```python
from build123d import *

# Parameters (mm, degrees)
ESBO_O1_R                = 2.95
RESSALTO_EXTRUS_O1_DEPTH = 16.15
RESSALTO_EXTRUS_O2_DEPTH = 32.3
FILETE1_R                = 1.5
ESBO_O3_R                = 3.25
CORTE_EXTRUS_O1_DEPTH    = 21.540435635
ESBO_O5_R                = 3.25
ESBO_O5_R_2              = 2.1
RESSALTO_EXTRUS_O3_DEPTH = 9.1
CHANFRO1_SIZE            = 1.2
ESBO_O7_R                = 2.875
RESSALTO_EXTRUS_O6_DEPTH = 15
FILETE2_R                = 2.5


with BuildPart() as part:
    # Esboço1 → Ressalto-extrusão1 (new, symmetric)
    with BuildSketch(Plane(origin=(0, 0, 0), x_dir=(0, 0, -1), z_dir=(1, 0, 0))):
        with BuildLine():
            Line((5.15, -6.450193796), (-5.15, -6.450193796))
            Line((-5.15, -6.450193796), (-5.15, 0))
            ThreePointArc((-5.15, 0), (0, 5.15), (5.15, 0))
            Line((5.15, 0), (5.15, -6.450193796))
        make_face()
        Circle(ESBO_O1_R, mode=Mode.SUBTRACT)
    extrude(amount=RESSALTO_EXTRUS_O1_DEPTH, both=True)

    # Esboço2 → Ressalto-extrusão2 (add, through all)
    with BuildSketch(Plane.ZY.offset(16.15)):
        with BuildLine():
            Line((-5.15, 0), (-5.15, -6.450193796))
            Line((-5.15, -6.450193796), (5.15, -6.450193796))
            Line((5.15, -6.450193796), (5.15, 0))
            ThreePointArc((5.15, 0), (0, 5.15), (-5.15, 0))
        make_face()
    extrude(amount=-RESSALTO_EXTRUS_O2_DEPTH)

    # Filete1
    filete1_edges = [part.edges().sort_by_distance(p)[0] for p in [
        (-16.15, -3.225096898, -5.15),
        (-16.15, -3.225096898, 5.15),
        (-16.15, 5.15, 0),
    ]]
    fillet(filete1_edges, radius=FILETE1_R)

    # Esboço3 → Corte-extrusão1 (cut, through all)
    with BuildSketch(Plane.XZ.offset(6.450193796)):
        with Locations(Location((-5.15, 0, 0), (0, 0, 270))):
            Circle(ESBO_O3_R)
        with Locations(Location((7.85, 0, 0), (0, 0, 270))):
            Circle(ESBO_O3_R)
    extrude(amount=-CORTE_EXTRUS_O1_DEPTH, mode=Mode.SUBTRACT)

    # Esboço5 → Ressalto-extrusão3 (add)
    # profile 1 of 2: a face of its own
    with BuildSketch(Plane.XZ.offset(6.450193796)):
        with Locations(Location((7.85, 0, 0), (0, 0, 270))):
            Circle(ESBO_O5_R)
        with Locations(Location((7.85, 0, 0), (0, 0, 270))):
            Circle(ESBO_O5_R_2, mode=Mode.SUBTRACT)
    # profile 2 of 2: a face of its own
    with BuildSketch(Plane.XZ.offset(6.450193796)):
        with Locations(Location((-5.15, 0, 0), (0, 0, 270))):
            Circle(ESBO_O5_R)
        with Locations(Location((-5.15, 0, 0), (0, 0, 270))):
            Circle(ESBO_O5_R_2, mode=Mode.SUBTRACT)
    extrude(amount=-RESSALTO_EXTRUS_O3_DEPTH)

    # Chanfro1
    # the kernel refuses this chamfer: 1.2 mm, written as the material it takes off along each edge
    with BuildSketch(Plane(origin=(-5.15, 2.649806204, 0), x_dir=(0, 0, -1), z_dir=(-1, 0, 0))) as chanfro1_piece_1_section:
        Polygon((2.1 + CHANFRO1_SIZE, 0), (2.1, CHANFRO1_SIZE), (2.1, 0), align=None)
    chanfro1_piece_1 = revolve(axis=Axis((-5.15, 2.649806204, 0), (0, -1, 0)), mode=Mode.PRIVATE)
    chanfro1_piece_1 = chanfro1_piece_1 & Plane(origin=(-5.15, 2.024165302, 0), x_dir=(0, 0, -1), z_dir=(0, -1, 0)) * Cylinder(3.25, 14, mode=Mode.PRIVATE)
    add(chanfro1_piece_1, mode=Mode.SUBTRACT)
    with BuildSketch(Plane(origin=(7.85, 2.649806204, 0), x_dir=(0, 0, -1), z_dir=(-1, 0, 0))) as chanfro1_piece_2_section:
        Polygon((2.1 + CHANFRO1_SIZE, 0), (2.1, CHANFRO1_SIZE), (2.1, 0), align=None)
    chanfro1_piece_2 = revolve(axis=Axis((7.85, 2.649806204, 0), (0, -1, 0)), mode=Mode.PRIVATE)
    chanfro1_piece_2 = chanfro1_piece_2 & Plane(origin=(7.85, 2.024165302, 0), x_dir=(0, 0, -1), z_dir=(0, -1, 0)) * Cylinder(3.25, 14, mode=Mode.PRIVATE)
    add(chanfro1_piece_2, mode=Mode.SUBTRACT)

    # Esboço7 → Ressalto-extrusão6 (add)
    with BuildSketch(Plane(origin=(16.15, 0, 0), x_dir=(0, 0, -1), z_dir=(1, 0, 0))):
        Circle(ESBO_O7_R)
    extrude(amount=RESSALTO_EXTRUS_O6_DEPTH)

    # Filete2
    filete2_edges = [part.edges().sort_by_distance(p)[0] for p in [
        (31.15, 0, 2.875),
    ]]
    fillet(filete2_edges, radius=FILETE2_R)


solid = part.part
```
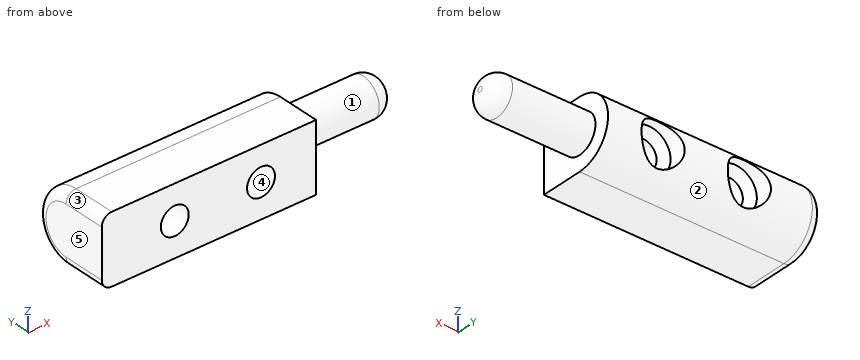
The listing builds one solid part. Answer for the finished solid, in the listing's coordinates (mm). Face numbers are marked on the shaded views. A direction names the side the tool comes from. Round coordinates to 2 decimals unless told otherwise and drop trailing zeros. Loops run counter-clockwise (first coordinate to the right, second up) from the corner with the lowest first, then second, coordinate; pieces in that order, holes last.
1) A cutting plane is placed at B-B on y = -2. Give the number of separate pieces and of enclosed holes in the cut face, plus the area to 3 significant figures.
Outcome:
separate pieces: 1
enclosed holes: 2
area: 362 mm2
2) Consider line 1 (X direction, y = -0.25, z = 0); line 2 (X direction, y = -4.75, z = 0); line 3 (Y direction, x = 4, z = -4). Determine where each line is inside the solid, lowest interval first.
Outcome:
line 1: x = -16.15 to -7.25, -3.05 to 5.75, 9.95 to 31.15
line 2: x = -16.15 to -7.25, -3.05 to 5.75, 9.95 to 16.15
line 3: y = -6.45 to 3.24
3) Given P1, Ø6, axis at x = 16.5, z = -3, coming from the +Y side; P2, Ø1.5, axis at y = -2, z = 1, coming from the +X side; P3, Ø1.5, axis at x = -5.5, z = -1, coming from the -Y side; P4, Ø1, axis at x = -5, y = 4, coming from the -Z side, each flat-ended and moving along its own axis, determine where each tip first touches the part or whether it passes through.
Outcome:
P1: stops at y = 5.15
P2: stops at x = 30.89
P3: passes through
P4: stops at z = -3.78
4) A cutting plane is placed at A-A on x = -5.15. Determine the outline of the cut face in (y, z) (3 decimals), plus the area to 3 significant figures.
Outcome:
outline: (-6.45, -5.15) - (0, -5.15) arc R5.15 ccw to (3.995, -3.25) - (2.6, -3.25) - (1.45, -2.1) - (-6.45, -2.1) - close; (-6.45, 2.1) - (1.45, 2.1) - (2.6, 3.25) - (3.995, 3.25) arc R5.15 ccw to (0, 5.15) - (-6.45, 5.15) - close
area: 54.6 mm2
5) For the marked faces 1 and 2, determine the directions among +Z, -Z, +X, -X, +Y, -Y from which every point of the face is accessible in a straight line to the end or side of a thin tool.
Outcome:
face 1: +X
face 2: +X, -X, +Y
6) A cutting plane is placed at D-D on x = 23.5. Determine the outline of the cut face in (y, z) (3 decimals).
Outcome:
outline: circle Ø5.75 at (0, 0)
7) A cutting plane is placed at C-C on x = 3.5. Determine the outline of the cut face in (y, z).
Outcome:
outline: (-6.45, -5.15) - (0, -5.15) arc R5.15 ccw to (0, 5.15) - (-6.45, 5.15) - close
8) For a pull along Z with two mould halves and no side action, classify the marked faces 3, 4 and 5 as released by +Z, released by -Z, zero draft, split by the parting line, or undercut.
Outcome:
face 3: released by +Z
face 4: undercut
face 5: zero draft
